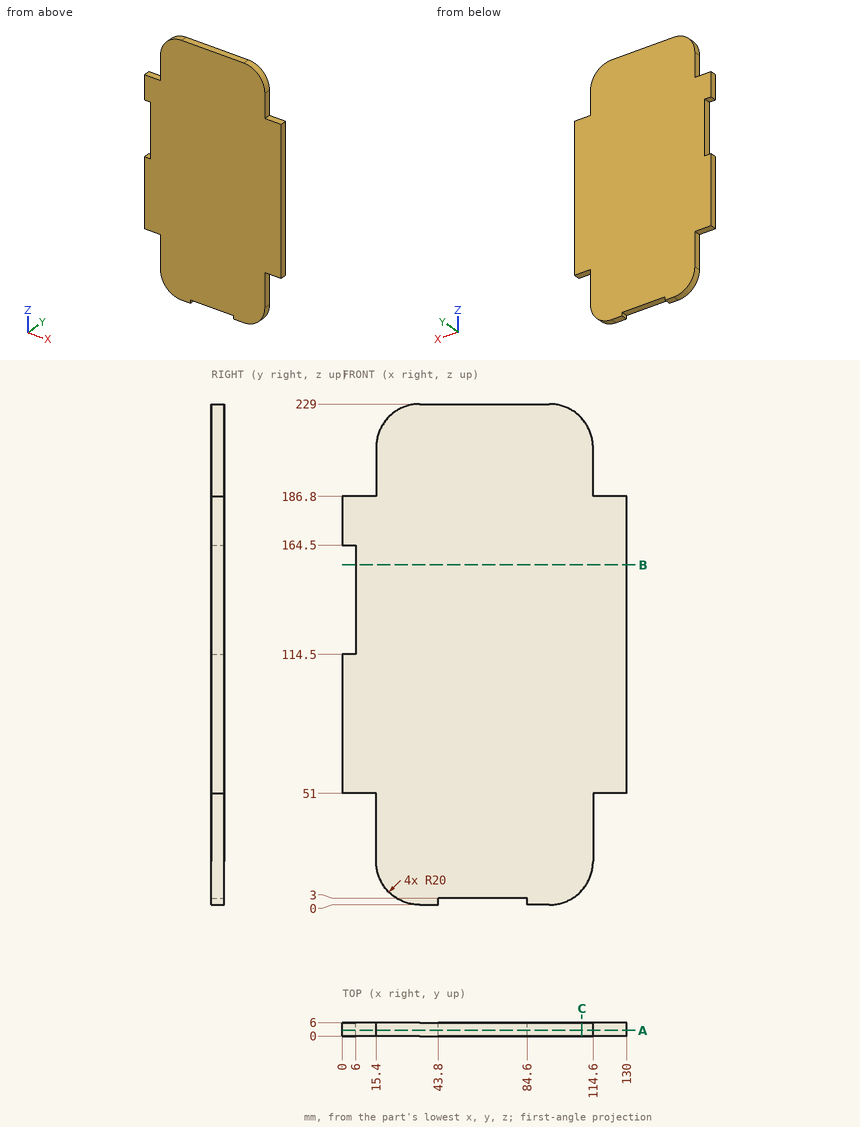
Verification items for this drawing (mm, ordinates from the low corner). Round coordinates to 2 decimals unless told otherwise and drop trailing zeros. Order: outer loops, then holes, each group sorted by start corner. A loop starts at its lowest first (then second) coordinate and runs counter-clockwise, first axis right, second up. Notation, with made-up numbers: (-4, 25.5) - (36, 25.5) arc R29 ccw to (36, 46.5) - close; hole circle Ø8 at (75, 22). An arc over 180 degrees is marked (long way). Answer as CSV lines item,"result". Start each with the question number.
1) Section check A-A (y = 2.6). Record the cut outline in (x, z), then the cut area to 3 significant figures.
2) Scan lines: probe 1 along Z at (x, y) = (115.5, 1.3); probe 2 along X at (y, z) = (0.55, 31.5); probe 3 along Z at (x, y) = (78, 3.5). Record each from-to range of solid material in increasing order.
3) Section check B-B (z = 155.5). Record the cut outline in (x, y), then the cut area to 3 significant figures.
4) Section check C-C (x = 109.5). Record the cut outline in (y, z), then the cut area to 3 significant figures.
5) Depth check by flat-ended pin: pin 1 (1.8 mm diameter, centred on y = 1.5, z = 39.5, fed in from -X); pin 2 (3.5 mm diameter, centred on y = 4.5, z = 2, fed in from +X); pin 3 (3 mm diameter, centred on x = 8, y = 2, fed in from -Z). Enter the tip coordinate at first touch or a pass-through.
Determined:
1,outline,"(0, 51) - (15.4, 51) - (15.4, 20) arc R20 ccw to (35.4, 0) - (43.8, 0) - (43.8, 3) - (84.6, 3) - (84.6, 0) - (94.6, 0) arc R20 ccw to (114.6, 20) - (114.6, 51) - (130, 51) - (130, 186.8) - (114.6, 186.8) - (114.6, 209) arc R20 ccw to (94.6, 229) - (35.4, 229) arc R20 ccw to (15.4, 209) - (15.4, 186.8) - (0, 186.8) - (0, 164.5) - (6, 164.5) - (6, 114.5) - (0, 114.5) - close"
1,area,"26,100 mm^2"
2,probe 1,"51 to 186.8"
2,probe 2,"15.4 to 114.6"
2,probe 3,"3 to 229"
3,outline,"(6, 0) - (130, 0) - (130, 6) - (6, 6) - close"
3,area,"744 mm^2"
4,outline,"(0, 6.66) - (6, 6.66) - (6, 222.34) - (0, 222.34) - close"
4,area,"1,290 mm^2"
5,pin 1,"x = 15.4"
5,pin 2,"x = 106.26"
5,pin 3,"z = 51"
